CAD build for the part. Positions are in the model's coordinates, mm. A direction names the side the tool comes from. Round coordinates to 2 decimals unless told otherwise and drop trailing zeros. Loops run counter-clockwise (first coordinate to the right, second up) from the corner with the lowest first, then second, coordinate; pieces in that order, holes last. Notation, with made-up numbers: M 31.5,4.5 L 80.5,4.5 A34 ccw 80.5,39.5 Z; hole C -34.5,61.25 d8. An arc over 180 degrees is marked long. Use a Markdown table: item, result. Add a question column.
(1) Flat gauge pins, fed straight in: P1, Ø12, axis at y = 6, z = 10.5, coming from the +X side; P2, Ø1.5, axis at x = 3.5, y = -12.5, coming from the -Z side; P3, Ø9, axis at x = 6.5, y = 0.5, coming from the +Z side; P4, Ø5, axis at x = 8.57, y = -9.52, coming from the -Z side. Where does each tip first touch, or does it go through?
(2) Two-plate mould, pull along Y, no slides. Class faces 3 (the face through (1, -19.05, 6)), 4 (the face through (20, 0, 1)), 5 (the face through (0.74, -11.23, 11.25)): released by +Y, released by -Y, zero draft, split by the parting line, or undercut.
(3) Band-saw the part on A-A, the plane y = -7.5. Write the cut outline in (x, z).
(4) Which spindle directions (+Z, -Z, +X, -X, +Y, -Y) get a long thin tool onto all of the face, cutting with end or side? Do faces 1 (the face through (0.74, 11.523, 5.803)), 2 (the face through (1.5, 0, 11)). Say none if no direction does.
(5) Wall check: L1, parallel to Z at x = 3, y = 1.5; L2, parallel to Y at x = 11, z = 1.25. Give the ranges that are in metal, low to high.
(6) Band-saw the part on B-B, the plane z = 10. Write the cut outline in (x, y), and give its area (3 significant figures).
(7) Band-saw the part on C-C, the plane y = 16. Write the cut outline in (x, z), and give its area (3 significant figures).
(8) Band-saw the part on D-D, the plane x = 14. Write the cut outline in (y, z), and give its area (4 significant figures).
from build123d import *

# Parameters (mm, degrees)
F1_DEPTH = 19.05
F2_R     = 3.175
F2_R_2   = 2
F3_DEPTH = 1.5
F4_R     = 3.175
F4_R_2   = 2
F5_DEPTH = 1.5


with BuildPart() as f1:
    # F0 (on Front) → F1 (new body, symmetric)
    with BuildSketch(Plane.XZ):
        with BuildLine():
            Line((1.5, 20), (0, 20))
            Line((0, 20), (0, 0))
            Line((0, 0), (20, 0))
            Line((20, 0), (20, 1.5))
            Line((20, 1.5), (1.754, 1.5))
            ThreePointArc((1.754, 1.5), (1.574395, 1.574395), (1.5, 1.754))
            Line((1.5, 1.754), (1.5, 20))
        make_face()
    extrude(amount=F1_DEPTH, both=True)

    # F2 (on face) → F3 (cut, through all)
    with BuildSketch(Plane(origin=(0, 0, 0), x_dir=(0, -1, 0), z_dir=(-1, 0, 0))):
        with Locations((9.525, 8.5725)):
            Circle(F2_R)
        with Locations((-9.525, 5.715)):
            Circle(F2_R_2)
    extrude(amount=-F3_DEPTH, mode=Mode.SUBTRACT)

    # F4 (on face) → F5 (cut, through all)
    with BuildSketch(Plane(origin=(0, 0, 0), x_dir=(1, 0, 0), z_dir=(0, 0, -1))):
        with Locations((8.5725, 9.525)):
            Circle(F4_R)
        with Locations((5.715, -9.525)):
            Circle(F4_R_2)
    extrude(amount=-F5_DEPTH, mode=Mode.SUBTRACT)


solid = f1.part
Return value:
| question | item | result |
|---|---|---|
| 1 | P1 | x = 1.5 |
| 1 | P2 | z = 0 |
| 1 | P3 | z = 1.5 |
| 1 | P4 | through |
| 2 | face 3 | released by -Y |
| 2 | face 4 | zero draft |
| 2 | face 5 | undercut |
| 3 | outline | M 0,0 L 6.13,0 L 6.13,1.5 L 1.75,1.5 A0.25 cw 1.5,1.75 L 1.5,6.13 L 0,6.13 Z; M 0,11.02 L 1.5,11.02 L 1.5,20 L 0,20 Z; M 11.02,0 L 20,0 L 20,1.5 L 11.02,1.5 Z |
| 4 | face 1 | +X, -X |
| 4 | face 2 | +Z, +X, +Y, -Y |
| 5 | L1 | 0 to 1.5 |
| 5 | L2 | -19.05 to -11.57, -7.48 to 19.05 |
| 6 | outline | M 0,-19.05 L 1.5,-19.05 L 1.5,-12.36 L 0,-12.36 Z; M 0,-6.69 L 1.5,-6.69 L 1.5,19.05 L 0,19.05 Z |
| 6 | area | 48.6 mm^2 |
| 7 | outline | M 0,0 L 20,0 L 20,1.5 L 1.75,1.5 A0.25 cw 1.5,1.75 L 1.5,20 L 0,20 Z |
| 7 | area | 57.8 mm^2 |
| 8 | outline | M -19.05,0 L 19.05,0 L 19.05,1.5 L -19.05,1.5 Z |
| 8 | area | 57.15 mm^2 |
